Read the model definition and answer for the solid it produces. Units are mm, in the model's axes. Face numbers are marked on the shaded views. A direction names the side the tool comes from. Give positions to 0.01 mm unless a question says otherwise; leave off trailing zeros. Write each loop counter-clockwise with the first axis right and the second up, starting at its lowest first coordinate (ties: lowest second). Pieces come first, ordered by that corner, then holes. Notation, with made-up numbers: M 55,-39 L 104,-39 A21 cw 104,-17 Z; hole C 44,58 d8. An arc over 180 degrees is marked long. Answer as CSV lines item,"result". Start each with the question number.
```python
from build123d import *

# Parameters (mm, degrees)
BOSS_EXTRUDE1_DEPTH     = 4
CHAMFER1_SIZE           = 3
CUT_EXTRUDE1_DEPTH      = 45.833023543
CUT_EXTRUDE1_DEPTH_BACK = 45.833023543
SKETCH3_R               = 1.55
FILLET1_R               = 4


with BuildPart() as part:
    # Sketch1 → Boss-Extrude1 (new, symmetric)
    with BuildSketch(Plane(origin=(0, 0, 0), x_dir=(1, 0, 0), z_dir=(0, 1, 0))):
        Polygon((-25, 37), (25, 37), (25, 33), (15, 33), (15, -33), (25, -33), (25, -37), (-25, -37), (-25, -33), (-15, -33), (-15, 33), (-25, 33), align=None)
        with BuildLine():
            Line((-5, -17.5), (-5, 17.5))
            ThreePointArc((-5, 17.5), (0, 22.5), (5, 17.5))
            Line((5, 17.5), (5, -17.5))
            ThreePointArc((5, -17.5), (0, -22.5), (-5, -17.5))
        make_face(mode=Mode.SUBTRACT)
    extrude(amount=BOSS_EXTRUDE1_DEPTH, both=True)

    # Chamfer1
    chamfer1_edges = [part.edges().sort_by_distance(p)[0] for p in [
        (-15, 0, 33),
        (-15, 0, -33),
        (15, 0, -33),
        (15, 0, 33),
    ]]
    chamfer(chamfer1_edges, length=CHAMFER1_SIZE)

    # Sketch3 → Cut-Extrude1 (cut, two sides: drawn at the far end of the back side and taken through both)
    with BuildSketch(Plane.XY.offset(-CUT_EXTRUDE1_DEPTH_BACK)):
        with Locations((-21, 0)):
            Circle(SKETCH3_R)
        with Locations(Location((21, 0, 0), (0, 0, 180))):
            Circle(SKETCH3_R)
    extrude(amount=CUT_EXTRUDE1_DEPTH + CUT_EXTRUDE1_DEPTH_BACK, mode=Mode.SUBTRACT)

    # Fillet1
    fillet1_edges = [part.edges().sort_by_distance(p)[0] for p in [
        (25, -4, 35),
        (-25, -4, 35),
        (-25, 4, 35),
        (25, 4, 35),
        (25, -4, -35),
        (25, 4, -35),
        (-25, -4, -35),
        (-25, 4, -35),
    ]]
    fillet(fillet1_edges, radius=FILLET1_R - 0.0001)  # a hair under: the kernel refuses the full size


solid = part.part
```
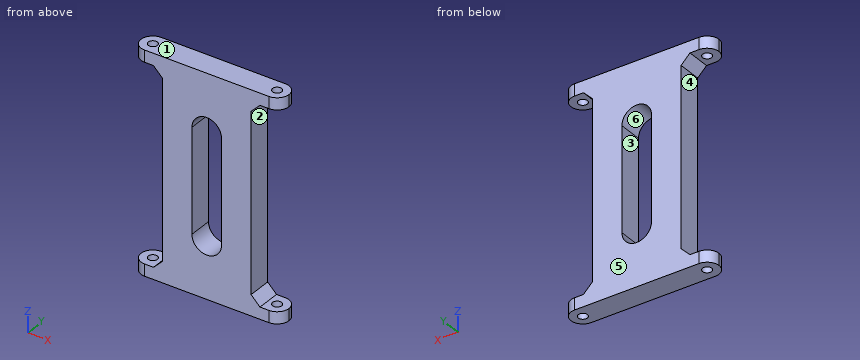
1. Find the intervals of material crossed by line 1 (Y direction, x = -21, z = 35.8); line 2 (X direction, y = 3, z = -4.5); line 3 (Z direction, x = 16.5, y = 2.25), in increasing order. Write a range as [from, to].
2. Determine the mould class of the marked faces 4, 5 and 6 for opening direction X: +X half, -X half, draft (parallel to the pull), parting line (faces both ways), or undercut.
3. Find section B-B on x = 0. Determine the outline of the cut face in (y, z).
4. For the marked faces 1, 2 and 3, determine the directions among +Z, -Z, +X, -X, +Y, -Y from which every point of the face is accessible in a straight line to the end or side of a thin tool.
5. Given pin 1 (1.5 mm diameter, centred on y = -3, z = 23, fed in from +X); pin 2 (4 mm diameter, centred on y = 2, z = 0.5, fed in from -X); pin 3 (4 mm diameter, centred on x = -1.5, z = -5, fed in from +Y), each flat-ended and moving along its own axis, determine where each tip first touches the part or whether it passes through.
6. Find section C-C on y = -2.75. Determine the outline of the cut face in (x, z).
7. Find section A-A on z = -21.5. Determine the outline of the cut face in (x, y).
Computed:
1,line 1,"y = [-4, -1.55], [1.55, 4]"
1,line 2,"x = [-15, -5], [5, 15]"
1,line 3,"z = [-37, -31.5], [31.5, 37]"
2,face 4,"-X half"
2,face 5,"draft"
2,face 6,"undercut"
3,outline,"M -4,-37 L 4,-37 L 4,-22.5 L -4,-22.5 Z; M -4,22.5 L 4,22.5 L 4,37 L -4,37 Z"
4,face 1,"+Z, +X, -X, +Y, -Y"
4,face 2,"+X, +Y, -Y"
4,face 3,"+Y, -Y"
5,pin 1,"stops at x = 15"
5,pin 2,"stops at x = -15"
5,pin 3,"passes through"
6,outline,"M -23.9,-37 L 23.9,-37 L 23.9,-33 L 18,-33 L 15,-30 L 15,30 L 18,33 L 23.9,33 L 23.9,37 L -23.9,37 L -23.9,33 L -18,33 L -15,30 L -15,-30 L -18,-33 L -23.9,-33 Z; hole M -5,-17.5 A5 ccw 5,-17.5 L 5,17.5 A5 ccw -5,17.5 Z"
7,outline,"M -15,-4 L -3,-4 L -3,4 L -15,4 Z; M 3,-4 L 15,-4 L 15,4 L 3,4 Z"
